```python
from build123d import *

# Parameters (mm, degrees)
BOSS_EXTRUDE1_DEPTH = 10
SKETCH2_R           = 2.6
CUT_EXTRUDE4_DEPTH  = 25
CUT_EXTRUDE5_DEPTH  = 10
SKETCH6_R           = 4.5
CUT_EXTRUDE6_DEPTH  = 2
BOSS_EXTRUDE2_START = 1
SKETCH7_W           = 18
SKETCH7_H           = 10
SKETCH7_R           = 2.1
BOSS_EXTRUDE2_DEPTH = 1


with BuildPart() as part:
    # Sketch1 → Boss-Extrude1 (new body)
    with BuildSketch(Plane.XY):
        Polygon((-6, 0), (6, 0), (6, 22), (9, 22), (9, -3), (-9, -3), (-9, 22), (-6, 22), align=None)
    extrude(amount=BOSS_EXTRUDE1_DEPTH)

    # Sketch2 → Cut-Extrude4 (cut)
    with BuildSketch(Plane.ZY.offset(9)):
        with Locations((5, 16)):
            Circle(SKETCH2_R)
    extrude(amount=-CUT_EXTRUDE4_DEPTH, mode=Mode.SUBTRACT)

    # Sketch5 → Cut-Extrude5 (cut)
    with BuildSketch(Plane.XZ.offset(3)):
        with BuildLine():
            Line((2.1, 5), (0, 5))
            Line((0, 5), (-2.1, 5))
            ThreePointArc((-2.1, 5), (0, 2.9), (2.1, 5))
        make_face()
        with BuildLine():
            Line((0, 7.1), (0, 5))
            Line((0, 5), (2.1, 5))
            ThreePointArc((2.1, 5), (1.48492424, 6.48492424), (0, 7.1))
        make_face()
        with BuildLine():
            Line((-2.1, 5), (0, 5))
            Line((0, 5), (0, 7.1))
            ThreePointArc((0, 7.1), (-1.48492424, 6.48492424), (-2.1, 5))
        make_face()
    extrude(amount=-CUT_EXTRUDE5_DEPTH, mode=Mode.SUBTRACT)

    # Sketch6 → Cut-Extrude6 (cut)
    with BuildSketch(Plane(origin=(0, 0, 0), x_dir=(1, 0, 0), z_dir=(0, 1, 0))):
        with Locations(Location((0, -5, 0), (0, 0, 180))):
            Circle(SKETCH6_R)
    extrude(amount=-CUT_EXTRUDE6_DEPTH, mode=Mode.SUBTRACT)

    # Sketch7 → Boss-Extrude2 (add)
    with BuildSketch(Plane.XZ.offset(3).offset(BOSS_EXTRUDE2_START)):
        with Locations((0, 5)):
            Rectangle(SKETCH7_W, SKETCH7_H)
        with Locations(Location((0, 5, 0), (0, 0, 270))):
            Circle(SKETCH7_R, mode=Mode.SUBTRACT)
    extrude(amount=-BOSS_EXTRUDE2_DEPTH)


solid = part.part
```
Read the model definition and answer for the solid it produces. Units are mm, in the model's axes. A direction names the side the tool comes from. Coordinates: 2 decimals unless noted, no trailing zeros. Loops run counter-clockwise (first coordinate to the right, second up) from the corner with the lowest first, then second, coordinate; pieces in that order, holes last.
(1) Flat-ended cylindrical pins translate along their axes: pin 1 Ø4 at (x, z) = (0, 5) entering from +Y; pin 2 Ø5 at (x, z) = (1.5, 5) entering from +Y. Find the tip coordinate at first contact, or state that the pin passes through.
Solution:
pin 1: passes through
pin 2: stops at y = -2
(2) The part is cut by section B-B (y = 16). Determine the outline of the cut face in (x, z), and give its area (3 significant figures).
Solution:
outline: (-9, 0) - (-6, 0) - (-6, 2.4) - (-9, 2.4) - close; (-9, 7.6) - (-6, 7.6) - (-6, 10) - (-9, 10) - close; (6, 0) - (9, 0) - (9, 2.4) - (6, 2.4) - close; (6, 7.6) - (9, 7.6) - (9, 10) - (6, 10) - close
area: 28.8 mm2
(3) The part is cut by section D-D (y = -1.25). Determine the outline of the cut face in (x, z), and give its area (3 significant figures).
Solution:
outline: (-9, 0) - (9, 0) - (9, 10) - (-9, 10) - close; hole circle Ø9 at (0, 5)
area: 116 mm2
(4) Consider line 1 along Z through (x, y) = (0, -2.7); line 2 along X through (y, z) = (-3.15, 5); line 3 along X through (y, z) = (4.75, 6.25). Determine where each line is inside the solid, lowest interval first.
Solution:
line 1: z = 0 to 2.9, 7.1 to 10
line 2: x = -9 to -2.1, 2.1 to 9
line 3: x = -9 to -6, 6 to 9
(5) A tool of negligible diameter and unlimited length cuts with its end or side. For faces 5 (the face through (7, 22, 5)), 6 (the face through (-6, 11, 5)), 7 (the face through (0.98, -0.99, 0.61)), from which of +Z, -Z, +X, -X, +Y, -Y can it reach the whole face along a straight path? Write none if from no direction.
Solution:
face 5: +Z, -Z, +X, -X, +Y
face 6: +Z, -Z, +Y
face 7: +Y
(6) The part is cut by section A-A (y = 20.5). Determine the outline of the cut face in (x, z).
Solution:
outline: (-9, 0) - (-6, 0) - (-6, 10) - (-9, 10) - close; (6, 0) - (9, 0) - (9, 10) - (6, 10) - close
(7) The mould has two halves that part along Z. Classify faces 1 (the face through (-8, 6, 10)), 2 (the face through (2.1, -2, 4.1)), 3 (the face through (-8, 22, 5)), 4 (the face through (-8, 6, 0)): released by +Z, released by -Z, zero draft, split by the parting line, or undercut.
Solution:
face 1: released by +Z
face 2: undercut
face 3: zero draft
face 4: released by -Z
